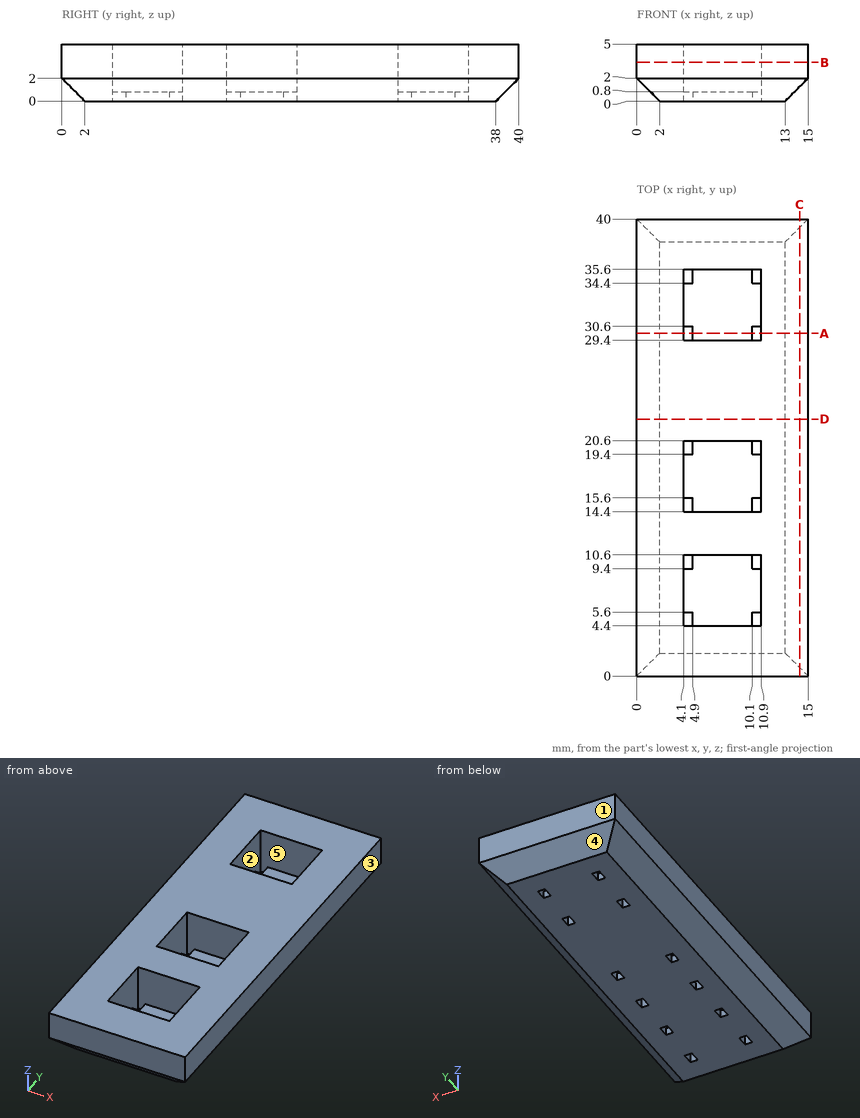
Job drawing, mm, ordinate dimensions from the low corner. One solid piece. A direction names the side the tool comes from. Give positions to 0.01 mm unless a question says otherwise; leave off trailing zeros. Write each loop counter-clockwise with the first axis right and the second up, starting at its lowest first coordinate (ties: lowest second). Pieces come first, ordered by that corner, then holes. Notation, with made-up numbers: (84, -16.5) - (88, -16.5) arc R19 ccw to (88, 0.5) - close; hole circle Ø2 at (22, 2.5). An arc over 180 degrees is marked (long way). Use one line per item in the form item = value. Start each with the question number.
1. Band-saw the part on A-A on y = 30. Write the cut outline in (x, z).
2. Band-saw the part on C-C on x = 14.25. Write the cut outline in (y, z).
3. Two-plate mould, pull along Y, no slides. Class the marked faces 1, 2 and 3: released by +Y, released by -Y, zero draft, split by the parting line, or undercut.
4. Probe line 1 (Y direction, x = 7.5, z = 3.15); line 2 (X direction, y = 18, z = 3.8); line 3 (Z direction, x = 9, y = 5). List the from-to ranges inside material, lowest first. Write a range as [from, to].
5. Band-saw the part on B-B on z = 3.4. Write the cut outline in (x, y), plus the area to 3 significant figures.
6. Band-saw the part on D-D on y = 22.5. Write the cut outline in (x, z), plus the area to 3 significant figures.
7. 3-axis set-ups, long thin cutter, end or side, ignore diameter. For the marked faces 4 and 5: which of +Z, -Z, +X, -X, +Y, -Y reach the whole face in a straight line?
8. Drop flat-ended pins along their axis: pin 1 Ø0.9 at (y, z) = (10, 0) entering from +X; pin 2 Ø0.6 at (x, z) = (4.5, 0.5) entering from +Y; pin 3 Ø0.6 at (x, z) = (4.5, 0) entering from -Y. Give the stop position or say it passes through.
Conclusion:
q1.outline = (0, 2) - (2, 0) - (4.1, 0) - (4.1, 5) - (0, 5) - close; (4.9, 0) - (10.1, 0) - (10.1, 0.8) - (4.9, 0.8) - close; (10.9, 0) - (13, 0) - (15, 2) - (15, 5) - (10.9, 5) - close
q2.outline = (0, 2) - (0.75, 1.25) - (39.25, 1.25) - (40, 2) - (40, 5) - (0, 5) - close
q3.face_1 = released by +Y
q3.face_2 = undercut
q3.face_3 = zero draft
q4.line_1 = [0, 4.4], [10.6, 14.4], [20.6, 29.4], [35.6, 40]
q4.line_2 = [0, 4.1], [10.9, 15]
q4.line_3 = [0, 0.8]
q5.outline = (0, 0) - (15, 0) - (15, 40) - (0, 40) - close; hole (4.1, 4.4) - (10.9, 4.4) - (10.9, 10.6) - (4.1, 10.6) - close; hole (4.1, 14.4) - (10.9, 14.4) - (10.9, 20.6) - (4.1, 20.6) - close; hole (4.1, 29.4) - (10.9, 29.4) - (10.9, 35.6) - (4.1, 35.6) - close
q5.area = 474 mm²
q6.outline = (0, 2) - (2, 0) - (13, 0) - (15, 2) - (15, 5) - (0, 5) - close
q6.area = 71.0 mm²
q7.face_4 = -Z, +X, -X, +Y
q7.face_5 = +Z
q8.pin_1 = 13.45
q8.pin_2 = 38.8
q8.pin_3 = 1.7
